```python
from build123d import *

# Parameters (mm, degrees)
BOSS_EXTRUDE1_DEPTH     = 5
SKETCH2_R               = 5
BOSS_EXTRUDE2_DEPTH     = 11
SKETCH3_W               = 30
SKETCH3_H               = 20
BOSS_EXTRUDE3_DEPTH     = 12
CUT_EXTRUDE1_DEPTH      = 26
CUT_EXTRUDE1_DEPTH_BACK = 6
SKETCH6_R               = 2.45
CUT_EXTRUDE2_DEPTH      = 5
FILLET1_R               = 0.3
FILLET2_R               = 5
FILLET3_R               = 0.5
SKETCH7_R               = 2.9
CUT_EXTRUDE3_DEPTH      = 6


with BuildPart() as part:
    # Sketch1 → Boss-Extrude1 (new body)
    with BuildSketch(Plane.XY):
        with BuildLine():
            ThreePointArc((10, 0), (0, 10), (-10, 0))
            ThreePointArc((-10, 0), (0, -10), (10, 0))
        make_face()
    extrude(amount=BOSS_EXTRUDE1_DEPTH)

    # Sketch2 → Boss-Extrude2 (add)
    with BuildSketch(Plane.XY):
        Circle(SKETCH2_R)
    extrude(amount=BOSS_EXTRUDE2_DEPTH)

    # Sketch3 → Boss-Extrude3 (add)
    with BuildSketch(Plane.XY.offset(11)):
        Rectangle(SKETCH3_W, SKETCH3_H)
    extrude(amount=BOSS_EXTRUDE3_DEPTH)

    # Sketch5 → Cut-Extrude1 (cut, two sides)
    with BuildSketch(Plane(origin=(-10, 0, 0), x_dir=(0, 0, -1), z_dir=(1, 0, 0))) as cut_extrude1_sk:
        Polygon((-23, 3.80444626), (-19.9, 5.25), (-19.9, -5.25), (-23, -3.80444626), align=None)
    extrude(amount=CUT_EXTRUDE1_DEPTH, mode=Mode.SUBTRACT)
    extrude(cut_extrude1_sk.sketch, amount=-CUT_EXTRUDE1_DEPTH_BACK, mode=Mode.SUBTRACT)

    # Sketch6 → Cut-Extrude2 (cut)
    with BuildSketch(Plane.XY.offset(23)):
        Circle(SKETCH6_R)
    extrude(amount=-CUT_EXTRUDE2_DEPTH, mode=Mode.SUBTRACT)

    # Fillet1
    fillet1_edges = [part.edges().sort_by_distance(p)[0] for p in [
        (0, 3.80444626, 23),
        (0, -3.80444626, 23),
        (0, -5.25, 19.9),
        (0, 5.25, 19.9),
    ]]
    fillet(fillet1_edges, radius=FILLET1_R)

    # Fillet2
    fillet2_edges = [part.edges().sort_by_distance(p)[0] for p in [
        (15, -10, 17),
        (15, 10, 17),
        (-15, 10, 17),
        (-15, -10, 17),
    ]]
    fillet(fillet2_edges, radius=FILLET2_R)

    # Fillet3
    fillet3_edges = [part.edges().sort_by_distance(p)[0] for p in [
        (-5, 0, 11),
        (10, 0, 0),
        (10, 0, 5),
        (-5, 0, 5),
    ]]
    fillet(fillet3_edges, radius=FILLET3_R)

    # Sketch7 → Cut-Extrude3 (cut)
    with BuildSketch(Plane.XY.offset(18)):
        Circle(SKETCH7_R)
    extrude(amount=-CUT_EXTRUDE3_DEPTH, mode=Mode.SUBTRACT)


solid = part.part
```
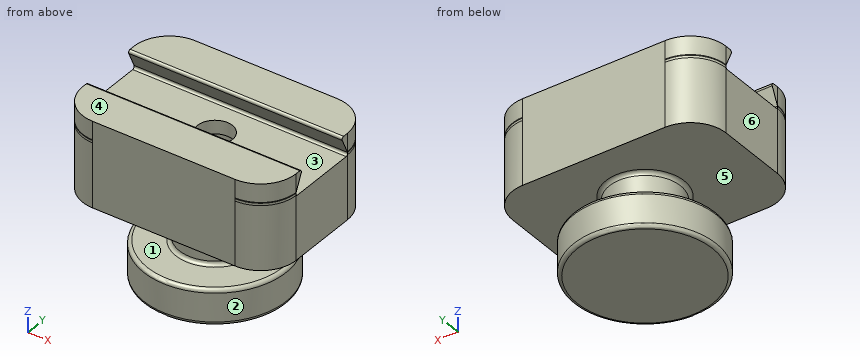
Geometry: final body of the model. Coordinates: model frame, mm. Face numbers are marked on the shaded views. A direction names the side the tool comes from. Give positions to 0.01 mm unless a question says otherwise; leave off trailing zeros. Order: outer loops, then holes, each group sorted by start corner. A loop starts at its lowest first (then second) coordinate and runs counter-clockwise, first axis right, second up. Notation, with made-up numbers: M 57.25,55.25 L 101.25,55.25 A23 cw 101.25,80.25 Z; hole C -15,71 d6. An arc over 180 degrees is marked long. Answer as CSV lines item,"result". Start each with the question number.
1) Cut plane B-B (y = 0). Output: boundary loops of the cut face in (x, z).
2) First-contact query: P1, Ø5, axis at y = -5, z = 2.5, coming from the -X side; P2, Ø6.5, axis at x = 0, y = 0, coming from the +Z side; P3, Ø12, axis at x = -11.5, z = 3.5, coming from the -Y side. Flat tips, straight axial feed; report the tip coordinate or a pass-through.
3) Cut plane C-C (z = 8.5). Output: boundary loops of the cut face in (x, y).
4) Cut plane A-A (z = 14). Output: boundary loops of the cut face in (x, y).
5) Mould query, pull axis Z, two halves, no side actions, for the marked faces 4, 5 and 6. Classes: +Z half, -Z half, draft (parallel to the pull), parting line (faces both ways), or undercut.
6) Set-up query: the marked faces 1, 2 and 3. Return all of +Z, -Z, +X, -X, +Y, -Y with unobstructed straight access to the full face (end or side cutting, diameter ignored); none if empty.
7) Line query: line 1 (Z direction, x = -5, y = -2.75); line 2 (Z direction, x = 1, y = 6.5); line 3 (Z direction, x = 7.5, y = -5). Output: solid intervals per line, ascending. Write a range as from..to.
Findings below:
1,outline,"M -15,11 L -5.5,11 A0.5 cw -5,10.5 L -5,5.5 A0.5 cw -5.5,5 L -9.5,5 A0.5 ccw -10,4.5 L -10,0.5 A0.5 ccw -9.5,0 L 9.5,0 A0.5 ccw 10,0.5 L 10,4.5 A0.5 ccw 9.5,5 L 5.5,5 A0.5 cw 5,5.5 L 5,10.5 A0.5 cw 5.5,11 L 15,11 L 15,19.9 L 2.45,19.9 L 2.45,18 L 2.9,18 L 2.9,12 L -2.9,12 L -2.9,18 L -2.45,18 L -2.45,19.9 L -15,19.9 Z"
2,P1,"stops at x = -9.68"
2,P2,"stops at z = 19.9"
2,P3,"stops at y = -8.35"
3,outline,"C 0,0 d10"
4,outline,"M -15,-5 A5 ccw -10,-10 L 10,-10 A5 ccw 15,-5 L 15,5 A5 ccw 10,10 L -10,10 A5 ccw -15,5 Z; hole C 0,0 d5.8"
5,face 4,"+Z half"
5,face 5,"undercut"
5,face 6,"draft"
6,face 1,"none"
6,face 2,"-Z"
6,face 3,"+X, -X"
7,line 1,"z = 0..5, 11..19.9"
7,line 2,"z = 0..5, 11..23"
7,line 3,"z = 0..5, 11..20, 20.44..23"
